from build123d import *

# Parameters (mm, degrees)
SKETCH1_R           = 1.53
SKETCH1_R_2         = 5.5
BOSS_EXTRUDE1_DEPTH = 3
SKETCH2_R           = 2.55
CUT_EXTRUDE1_DEPTH  = 10
SKETCH4_W           = 31
SKETCH4_H           = 3
BOSS_EXTRUDE2_DEPTH = 15
FILLET1_R           = 4
FILLET4_R           = 1


with BuildPart() as part:
    # Sketch1 → Boss-Extrude1 (new body)
    with BuildSketch(Plane.XY):
        with BuildLine():
            Line((0, -11), (11, -11))
            Line((11, -11), (31, -11))
            Line((31, -11), (31, 11))
            Line((31, 11), (11, 11))
            Line((11, 11), (0, 11))
            ThreePointArc((0, 11), (-11, 0), (0, -11))
        make_face()
        with Locations((0, 8)):
            Circle(SKETCH1_R, mode=Mode.SUBTRACT)
        with Locations((8, 0)):
            Circle(SKETCH1_R, mode=Mode.SUBTRACT)
        with Locations((0, -8)):
            Circle(SKETCH1_R, mode=Mode.SUBTRACT)
        with Locations((-8, 0)):
            Circle(SKETCH1_R, mode=Mode.SUBTRACT)
        Circle(SKETCH1_R_2, mode=Mode.SUBTRACT)
    extrude(amount=BOSS_EXTRUDE1_DEPTH)

    # Sketch2 → Cut-Extrude1 (cut)
    with BuildSketch(Plane.XY):
        with Locations((21, 5.5)):
            Circle(SKETCH2_R)
        with Locations(Location((21, -5.5, 0), (0, 0, 180))):
            Circle(SKETCH2_R)
    extrude(amount=CUT_EXTRUDE1_DEPTH, mode=Mode.SUBTRACT)

    # Sketch4 → Boss-Extrude2 (add)
    with BuildSketch(Plane.XY):
        with Locations((15.5, 12.5)):
            Rectangle(SKETCH4_W, SKETCH4_H)
    extrude(amount=BOSS_EXTRUDE2_DEPTH)

    # Fillet1
    # the kernel refuses this fillet: 4 mm, written as the material it adds along each edge
    with BuildSketch(Plane(origin=(0, 11, 0), x_dir=(0, 1, 0), z_dir=(0, 0, 1))) as fillet1_piece_1:
        with BuildLine():
            CenterArc((3.464285714, 3.972963475), FILLET1_R, 195.358885581, 67.975687163)
            ThreePointArc((-0.392857143, 2.913506549), (-0.098656701, 1.469936831), (0, 0))
            Line((0, 0), (3, 0))
        make_face()
    extrude(amount=3)

    # Fillet4
    # the kernel refuses this fillet: 1 mm, written as the material it adds along each edge
    with BuildSketch(Plane(origin=(0, 11, 3), x_dir=(-1, 0, 0), z_dir=(0, 1, 0))) as fillet4_piece_1_section:
        with BuildLine():
            CenterArc((FILLET4_R, FILLET4_R), FILLET4_R, 180, 90)
            Line((0, FILLET4_R), (0, 0))
            Line((0, 0), (FILLET4_R, 0))
        make_face()
    fillet4_piece_1 = extrude(amount=3, mode=Mode.PRIVATE)
    fillet4_piece_1 = fillet4_piece_1 - Plane(origin=(-3.972963475, 14.464285714, 3.249866194), x_dir=(0, 1, 0), z_dir=(0, 0, -1)) * Cylinder(4, 10, mode=Mode.PRIVATE)
    add(fillet4_piece_1)


solid = part.part
Can you work these out from the model? Positions are in its coordinate system, mm. A direction names the side the tool comes from. Give positions to 0.01 mm unless a question says otherwise; leave off trailing zeros. Loops run counter-clockwise (first coordinate to the right, second up) from the corner with the lowest first, then second, coordinate; pieces in that order, holes last. Notation, with made-up numbers: M 22.5,33.25 L 26.5,33.25 A32 ccw 26.5,67.25 Z; hole C -1,-2 d7. An arc over 180 degrees is marked long. One line per item, written item: value. Start each with the question number.
1) On a 3-axis mill with a long thin cutter (end or side, diameter ignored), from which of +Z, -Z, +X, -X, +Y, -Y can I reach the whole of each face in a straight line? I mean faces 5 (the face through (31, 5, 2)), 6 (the face through (0, 12, 9)), 7 (the face through (15, 11, 9)). Say none if no direction works.
2) Thinking about a two-plate mould opening in X: for faces 1 (the face through (-1.19, -5.37, 1.48)), 2 (the face through (-0.3, -9.5, 1.5)), 3 (the face through (-0.2, 12.1, 3.4)), 4 (the face through (14, 2, 0)), which applies, +X half, -X half, draft (parallel to the pull), parting line (faces both ways), or undercut?
3) If we section it at D-D, the plane x = 21: Write out the boundary of the cut face in (y, z), and give its area (3 significant figures).
4) If we section it at A-A, the plane x = 8: Write out the boundary of the cut face in (y, z), and give its area (3 significant figures).
5) If we section it at C-C, the plane z = 2.5: Write out the boundary of the cut face in (x, y).
6) I'm going to push flat-ended pins straight in: pin 1 (3 mm diameter, centred on x = 8, y = 0, fed in from +Z) (3 decimals); pin 2 (1.5 mm diameter, centred on y = 2, z = 2.5, fed in from -X); pin 3 (7 mm diameter, centred on x = 15.5, y = 2.5, fed in from +Z); pin 4 (3.5 mm diameter, centred on y = 12, z = 10.5, fed in from -X). Where does each tip first touch, or does it pass through?
7) If I drill on line 1 (Y direction, x = 21, z = 0.85); line 2 (Y direction, x = 23, z = 10); line 3 (X direction, y = 11.5, z = 9.75), over which ranges is the centre line in solid material (lowest first)? Write a range as [from, to].
8) If we section it at B-B, the plane y = 0: Write out the boundary of the cut face in (x, z), and give its area (3 significant figures).
Completed:
1. face 5: +Z, -Z, +X, +Y, -Y
1. face 6: +Z, -X, +Y, -Y
1. face 7: +Z, +X, -X, -Y
2. face 1: undercut
2. face 2: undercut
2. face 3: -X half
2. face 4: draft
3. outline: M -11,0 L -8.05,0 L -8.05,3 L -11,3 Z; M -2.95,0 L 2.95,0 L 2.95,3 L -2.95,3 Z; M 8.05,0 L 14,0 L 14,15 L 11,15 L 11,3 L 8.05,3 Z
3. area: 80.4 mm^2
4. outline: M -11,0 L -1.53,0 L -1.53,3 L -11,3 Z; M 1.53,0 L 14,0 L 14,15 L 11,15 L 11,3 L 1.53,3 Z
4. area: 102 mm^2
5. outline: M -2.91,10.61 A11 ccw 0,-11 L 31,-11 L 31,14 L 0,14 A4 cw Z; hole C -8,0 d3.06; hole C 0,0 d11; hole C 0,-8 d3.06; hole C 0,8 d3.06; hole C 8,0 d3.06; hole C 21,-5.5 d5.1; hole C 21,5.5 d5.1
6. pin 1: passes through
6. pin 2: stops at x = -10.93
6. pin 3: stops at z = 3
6. pin 4: stops at x = 0
7. line 1: y = [-11, -8.05], [-2.95, 2.95], [8.05, 14]
7. line 2: y = [11, 14]
7. line 3: x = [0, 31]
8. outline: M -11,0 L -9.53,0 L -9.53,3 L -11,3 Z; M -6.47,0 L -5.5,0 L -5.5,3 L -6.47,3 Z; M 5.5,0 L 6.47,0 L 6.47,3 L 5.5,3 Z; M 9.53,0 L 31,0 L 31,3 L 9.53,3 Z
8. area: 74.6 mm^2
